Answer from the drawing. Dimensions are ordinates in mm from the lowest x, y and z of the part. Coordinates: 2 decimals unless noted, no trailing zeros. Write each loop counter-clockwise with the first axis right and the second up, starting at its lowest first coordinate (ties: lowest second). Pieces come first, ordered by that corner, then holes.
(1) Section B-B on z = 0.45 is taken. State how many separate pieces and enclosed holes the cut face has, then the cut area to 3 significant figures.
(2) Section A-A on x = 26.5 is taken. Write down the section's boundary in (y, z).
(3) Given pin 1 (4 mm diameter, centred on x = 23, y = 7, fed in from -Z), flat-ended and moving along its own axis, determine where the tip first touches the part or whether it passes through.
(4) Find the intervals of material crossed by probe 1 along Y at (x, z) = (21, 0.85); probe 2 along Y at (x, z) = (16, 1.4), in increasing order.
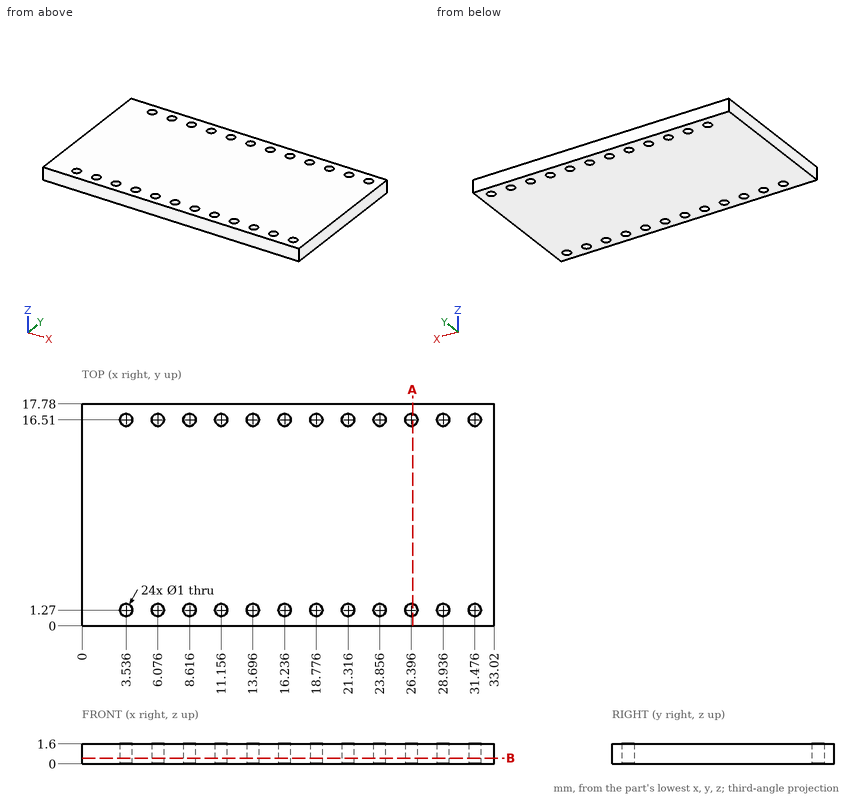
Response:
1. separate pieces: 1
1. enclosed holes: 24
1. area: 568 mm2
2. outline: (0, 0) - (0.78, 0) - (0.78, 1.6) - (0, 1.6) - close; (1.76, 0) - (16.02, 0) - (16.02, 1.6) - (1.76, 1.6) - close; (17, 0) - (17.78, 0) - (17.78, 1.6) - (17, 1.6) - close
3. pin 1: stops at z = 0
4. probe 1: y = 0 to 0.88, 1.66 to 16.12, 16.9 to 17.78
4. probe 2: y = 0 to 0.83, 1.71 to 16.07, 16.95 to 17.78
